The figure shows three views and two pictorial views of one solid part (mm, origin at its lowest corner). Answer the questions. A direction names the side the tool comes from. Coordinates: 2 decimals unless noted, no trailing zeros. Order: outer loops, then holes, each group sorted by start corner. A loop starts at its lowest first (then second) coordinate and runs counter-clockwise, first axis right, second up. Notation, with made-up numbers: (25.5, 78.5) -> (32.5, 78.5) arc R19 ccw to (32.5, 110.5) -> close; hole circle Ø2 at (70.25, 55.25). An arc over 180 degrees is marked (long way). Return JSON: item names as keys, results as strings. Group by question number.
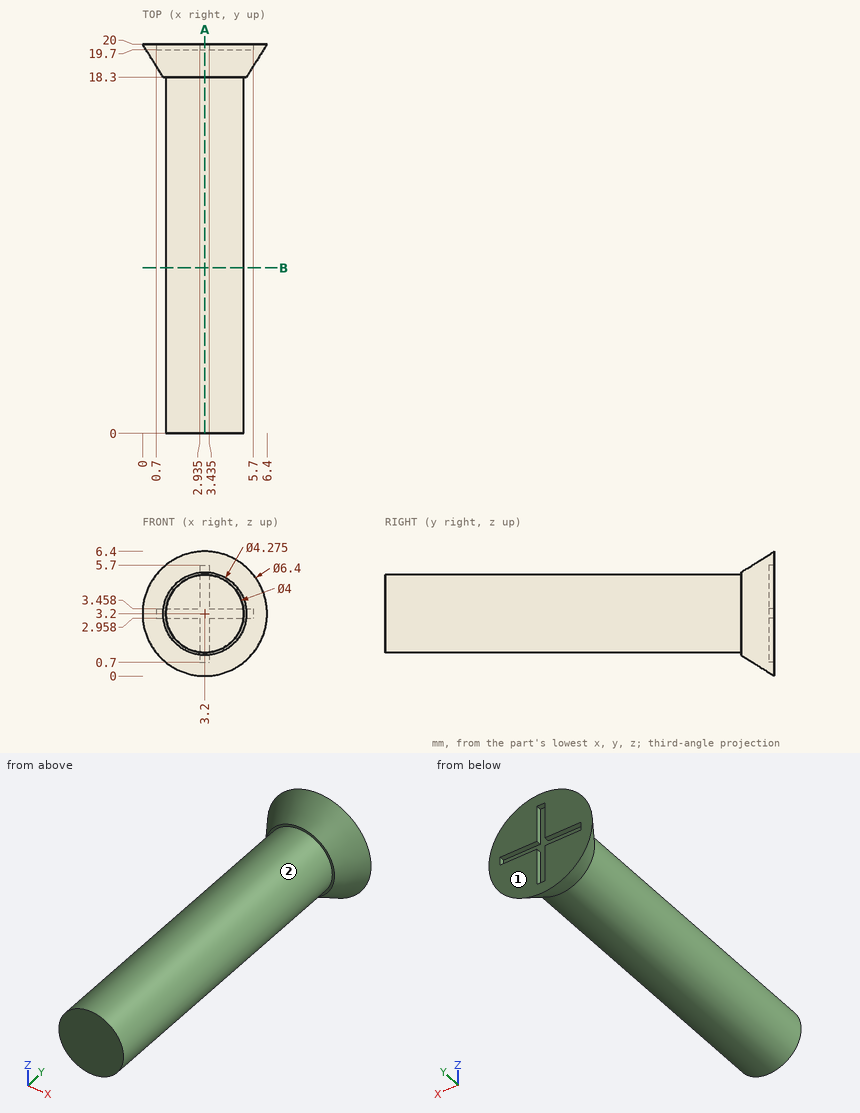
1. Find section A-A on x = 3.2. Determine the outline of the cut face in (y, z).
2. Given pin 1 (3 mm diameter, centred on y = 8.5, z = 3.5, fed in from +X); pin 2 (3 mm diameter, centred on x = 1.5, y = 2.5, fed in from -Z); pin 3 (1.3 mm diameter, centred on x = 2.5, z = 3, fed in from -Y); pin 4 (2 mm diameter, centred on x = 5, y = 5.5, fed in from -Z), each flat-ended and moving along its own axis, determine where each tip first touches the part or whether it passes through.
3. Which of the six approach directions +Z, -Z, +X, -X, +Y, -Y give full straight-line access (tool end or side, diameter ignored) to the marked faces 1 and 2?
4. Find section B-B on y = 8.5. Determine the outline of the cut face in (x, z).
5. Straight lines are drawn through the part: L1, parallel to Y at x = 5.25, z = 2.75; L2, parallel to Y at x = 3, z = 3; L3, parallel to X at y = 18.75, z = 1.75 (1 decimal). For each, find the intervals that lie inside material, in ascending order.
Result:
{
 "1": {"outline": "(0, 1.2) -> (18.3, 1.2) -> (18.3, 1.06) -> (20, 0) -> (20, 0.7) -> (19.7, 0.7) -> (19.7, 5.7) -> (20, 5.7) -> (20, 6.4) -> (18.3, 5.34) -> (18.3, 5.2) -> (0, 5.2) -> close"},
 "2": {"pin 1": "x = 5.2", "pin 2": "z = 1.21", "pin 3": "y = 0", "pin 4": "z = 1.37"},
 "3": {"face 1": "+Z, -Z, +X, -X, +Y", "face 2": "-Y"},
 "4": {"outline": "circle Ø4 at (3.2, 3.2)"},
 "5": {"L1": "18.3 to 20", "L2": "0 to 19.7", "L3": "1.3 to 5.1"}
}
